The model under review builds one solid part; all positions refer to its coordinate system, in mm. Face numbers are marked on the shaded views. A direction names the side the tool comes from. Round coordinates to 2 decimals unless told otherwise and drop trailing zeros. Write each loop counter-clockwise with the first axis right and the second up, starting at its lowest first coordinate (ties: lowest second). Pieces come first, ordered by that corner, then holes. Notation, with made-up numbers: (17.25, 77.25) - (31.25, 77.25) arc R10 cw to (31.25, 96.25) - close; hole circle Ø4 at (85.25, -34.5). An arc over 180 degrees is marked (long way). Use one line per item in the form item = value.
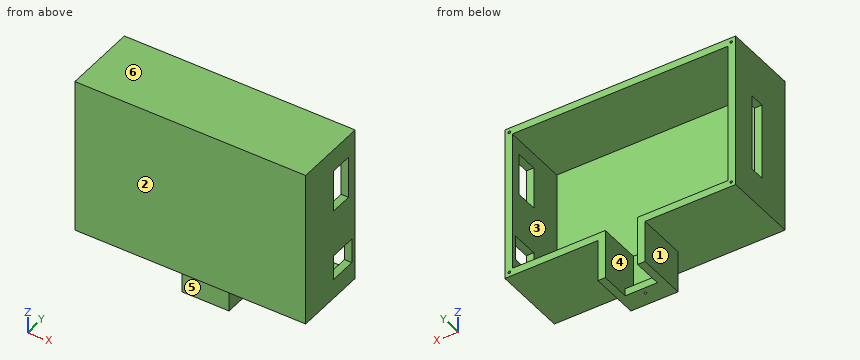
Autodesk Inventor part; units mm, degrees
ref_plane "YZ Plane" through (0, 0, 0) normal (1, 0, 0) x (0, 1, 0)
ref_plane "XZ Plane" through (0, 0, 0) normal (0, 1, 0) x (-1, 0, 0)
ref_plane "XY Plane" through (0, 0, 0) normal (0, 0, 1) x (1, 0, 0)
sketch "Sketch1" plane through (0, 0, 0) normal (0, 1, 0) x (-1, 0, 0)
  line L0 (46.5, 31.5) -> (-46.5, 31.5)
  line L1 (-46.5, 31.5) -> (-46.5, -31.5)
  line L2 (-46.5, -31.5) -> (46.5, -31.5)
  line L3 (46.5, -31.5) -> (46.5, 31.5)
  line L4 (46.5, 31.5) -> (-46.5, -31.5) construction
  line L5 (-46.5, 31.5) -> (46.5, -31.5) construction
  point P0 (0, 0)
  dimension "d0" = 63
  dimension "d1" = 93
extrude "Extrusion1" add sketch "Sketch1" along normal blind 3
sketch "Sketch2" plane through (0, 3, 0) normal (0, 1, 0) x (1, 0, 0)
  line L0 (-43.5, -28.5) -> (43.5, -28.5)
  line L1 (43.5, -28.5) -> (43.5, 28.5)
  line L2 (43.5, 28.5) -> (-43.5, 28.5)
  line L3 (-43.5, 28.5) -> (-43.5, -28.5)
  line L4 (-43.5, -28.5) -> (43.5, 28.5) construction
  line L5 (43.5, -28.5) -> (-43.5, 28.5) construction
  line L6 (46.5, -31.5) -> (46.5, 31.5)
  line L7 (-46.5, -31.5) -> (46.5, -31.5)
  line L8 (46.5, -31.5) -> (46.5, 31.5)
  line L9 (46.5, 31.5) -> (-46.5, 31.5)
  line L10 (-46.5, 31.5) -> (-46.5, -31.5)
  line L11 (-46.5, -31.5) -> (46.5, 31.5) construction
  line L12 (46.5, -31.5) -> (-46.5, 31.5) construction
  point P0 (0, 0)
  point P1 (46.5, -31.5)
  dimension "d4" = 57
  dimension "d5" = 87
extrude "Extrusion2" add sketch "Sketch2" along normal blind 27
sketch "Sketch3" plane through (0, 30, 0) normal (0, 1, 0) x (1, 0, 0)
  circle A0 centre (-44.7, 29.7) radius 0.5
  line L0 (46.5, 31.5) -> (-46.5, 31.5)
  line L1 (-46.5, 31.5) -> (-46.5, -31.5)
  circle A1 centre (-44.7, -29.7) radius 0.5
  line L2 (-46.5, -31.5) -> (46.5, -31.5)
  circle A2 centre (44.7, -29.7) radius 0.5
  line L3 (46.5, -31.5) -> (46.5, 31.5)
  circle A3 centre (44.7, 29.7) radius 0.5
  point P0 (0, 0)
  dimension "d8" = 1.8
  dimension "d9" = 1.8
  dimension "d10" = 1
  dimension "d11" = 1.8
  dimension "d12" = 1.8
  dimension "d13" = 1
  dimension "d14" = 1.8
  dimension "d15" = 1.8
  dimension "d16" = 1
  dimension "d17" = 1.8
  dimension "d18" = 1.8
  dimension "d19" = 1
extrude "Extrusion3" cut sketch "Sketch3" against normal blind 5 contours A0 | A1 | A2 | A3
sketch "Sketch5" plane through (-46.5, 0, -31.5) normal (-1, 0, 0) x (0, 0, 1)
  line L0 (13, 14) -> (44, 14)
  line L1 (44, 14) -> (44, 20)
  line L2 (44, 20) -> (13, 20)
  line L3 (13, 20) -> (13, 14)
  line L4 (0, 0) -> (63, 0)
  line L5 (0, 0) -> (0, 30)
  point P0 (31.5, 0)
  dimension "d23" = 14
  dimension "d24" = 6
  dimension "d25" = 31
  dimension "d26" = 13
extrude "Extrusion4" cut sketch "Sketch5" against normal blind 3
sketch "Sketch6" plane through (46.5, 0, 31.5) normal (1, 0, 0) x (0, 0, -1)
  line L0 (45, 28) -> (55, 28)
  line L1 (55, 28) -> (55, 17)
  line L2 (55, 17) -> (45, 17)
  line L3 (45, 17) -> (45, 28)
  line L4 (0, 0) -> (63, 0)
  line L5 (63, 0) -> (63, 30)
  line L6 (9, 26) -> (26, 26)
  line L7 (26, 26) -> (26, 17)
  line L8 (26, 17) -> (9, 17)
  line L9 (9, 17) -> (9, 26)
  line L10 (0, 0) -> (0, 30)
  point P0 (31.5, 0)
  dimension "d30" = 17
  dimension "d31" = 11
  dimension "d32" = 10
  dimension "d33" = 8
  dimension "d34" = 9
  dimension "d35" = 17
  dimension "d36" = 17
  dimension "d37" = 9
extrude "Extrusion5" cut sketch "Sketch6" against normal blind 3
sketch "Sketch7" plane through (46.5, 0, -31.5) normal (0, 0, -1) x (-1, 0, 0)
  line L0 (40.5, 41) -> (53.5, 41)
  line L1 (53.5, 41) -> (53.5, 13)
  line L2 (53.5, 13) -> (40.5, 13)
  line L3 (40.5, 13) -> (40.5, 41)
  line L4 (0, 0) -> (93, 0)
  line L5 (93, 0) -> (93, 30)
  point P0 (46.5, 0)
  dimension "d40" = 13
  dimension "d41" = 28
  dimension "d42" = 13
  dimension "d43" = 39.5
extrude "Extrusion6" cut sketch "Sketch7" against normal blind 3
sketch "Sketch8" plane through (46.5, 0, -31.5) normal (0, 0, -1) x (-1, 0, 0)
  line L0 (40.5, 30) -> (3, 30)
  line L1 (37.5, 30) -> (56.5, 30)
  line L2 (56.5, 30) -> (56.5, 10)
  line L3 (56.5, 10) -> (37.5, 10)
  line L4 (37.5, 10) -> (37.5, 30)
  line L5 (40.5, 13) -> (40.5, 30)
  line L6 (53.5, 30) -> (53.5, 13)
  line L7 (53.5, 13) -> (40.5, 13)
  point P0 (46.5, 0)
  dimension "d46" = 3
  dimension "d47" = 3
  dimension "d48" = 3
extrude "Extrusion7" add sketch "Sketch8" along normal blind 17 contours L5 L7 L6 L1 L2 L3 L4 L0
sketch "Sketch9" plane through (-7, 13, -28.5) normal (0, 1, 0) x (1, 0, 0)
  line L0 (13, 20) -> (13, 0)
  line L1 (0, 0) -> (0, 20)
  line L2 (13, 17) -> (0, 17)
  line L3 (0, 17) -> (0, 20)
  line L4 (0, 20) -> (13, 20)
  line L5 (13, 20) -> (13, 17)
  point P0 (7, -28.5)
  point P1 (0, 17)
  dimension "d51" = 3
extrude "Extrusion8" add sketch "Sketch9" along normal blind 5
sketch "Sketch10" plane through (46.5, 0, -48.5) normal (0, 0, -1) x (-1, 0, 0)
  circle A0 centre (47, 15.5) radius 0.5
  line L0 (40.5, 13) -> (53.5, 13)
  line L1 (40.5, 18) -> (40.5, 13)
  point P0 (46.5, 0)
  dimension "d54" = 2.5
  dimension "d55" = 6.5
  dimension "d56" = 1
extrude "Extrusion9" cut sketch "Sketch10" against normal blind 5
properties part number "remoteswitchbox"
(1) The part is to be moulded in two halves that separate along X. For the marked faces 1, 2 and 3, say which applies: +X half, -X half, draft (parallel to the pull), parting line (faces both ways), or undercut.
Geometry results:
face_1 = -X half
face_2 = draft
face_3 = undercut
(2) Machinability: for the marked faces 4, 5 and 6, which of the approach directions +Z, -Z, +X, -X, +Y, -Y give a long, thin tool a straight path to every point of the face, cutting with its end or side? Answer none if there is none.
Geometry results:
face_4 = +Y
face_5 = -Z, +X, -X, -Y
face_6 = +Z, +X, -X, +Y, -Y
(3) Insertion check: P1, Ø4, axis at x = -37, y = 13.5, coming from the -Z side; P2, Ø8.5, axis at x = -0.5, z = -43, coming from the -Y side; P3, Ø13.5, axis at y = 21.5, z = -38.5, coming from the -X side. Each pin has a flat end and moves straight along its axis. Give the tip position at first contact, or say it passes through.
Geometry results:
P1 = -31.5
P2 = 10
P3 = -10
(4) Add section A-A on z = -5. Write out the cut boundary in (x, y), then the cut area to 3 significant figures.
Geometry results:
outline = (-46.5, 0) - (46.5, 0) - (46.5, 30) - (43.5, 30) - (43.5, 3) - (-43.5, 3) - (-43.5, 14) - (-46.5, 14) - close; (-46.5, 20) - (-43.5, 20) - (-43.5, 30) - (-46.5, 30) - close
area = 423 mm2
(5) Add section B-B on y = 6.5. Write out the cut boundary in (x, z).
Geometry results:
outline = (-46.5, -31.5) - (46.5, -31.5) - (46.5, 31.5) - (-46.5, 31.5) - close; hole (-43.5, -28.5) - (43.5, -28.5) - (43.5, 28.5) - (-43.5, 28.5) - close
(6) Add section C-C on x = 2. Write out the cut boundary in (y, z), then the cut area to 3 significant figures.
Geometry results:
outline = (0, -31.5) - (10, -31.5) - (10, -48.5) - (18, -48.5) - (18, -45.5) - (13, -45.5) - (13, -28.5) - (3, -28.5) - (3, 28.5) - (30, 28.5) - (30, 31.5) - (0, 31.5) - close
area = 366 mm2
(7) To check wall thickness, follow L1, parallel to X at y = 28.7, z = 29.7; L2, parallel to X at y = 26.8, z = -29.7; L3, parallel to Z at x = -44.7, y = 26.2. State the ranges of each line that lie inside material, in increasing order.
Geometry results:
L1 = -46.5 to -45.2, -44.2 to 44.2, 45.2 to 46.5
L2 = -46.5 to -45.2, -44.2 to -7, 6 to 44.2, 45.2 to 46.5
L3 = -31.5 to -30.2, -29.2 to 29.2, 30.2 to 31.5
(8) Add section D-D on z = -25.5. Write out the cut boundary in (x, y).
Geometry results:
outline = (-46.5, 0) - (46.5, 0) - (46.5, 30) - (43.5, 30) - (43.5, 3) - (-43.5, 3) - (-43.5, 30) - (-46.5, 30) - close
